Geometry: final body of the model. Coordinates: model frame, mm. A direction names the side the tool comes from. Coordinates: 2 decimals unless noted, no trailing zeros. Loops run counter-clockwise (first coordinate to the right, second up) from the corner with the lowest first, then second, coordinate; pieces in that order, holes last. Notation, with made-up numbers: (88, 66) - (136, 66) arc R22 ccw to (136, 78) - close; hole circle Ø2 at (0.5, 6.25). An arc over 180 degrees is marked (long way). Put each result on its own line as item: value. Start each with the question number.
1) Section B-B on y = 45. Output: boundary loops of the cut face in (x, z), and give its area (3 significant figures).
2) Reachability of faces 5 (the cylindrical face through (38.315, -4.574, 3.614)), 6 (the cylindrical face through (40.354, 82.574, 5.325)), 7 (the cylindrical face through (-34.14, 4.9, 5.07)) from +Z, -Z, +X, -X, +Y, -Y: full face, straight path, thin tool, end or side. Return the list, or none.
3) Contact query for a flat-ended pin moving along its axis: pin 1 Ø2.5 at (x, z) = (-38.89, 5) entering from +Y. Output: stop coordinate, or through.
4) Section C-C on x = 6. Output: boundary loops of the cut face in (y, z).
5) Section D-D on y = 2. Output: boundary loops of the cut face in (x, z).
6) Material intervals for line 1 along X through (y, z) = (64, 7.25); line 2 along X through (y, z) = (82.15, 5); line 3 along Y through (x, z) = (9, 3.75), sorted ascending. Write a range as from..to.
7) Draft query along Z for faces 1 (the cylindrical face through (-44.4, -5.43, 5.07)), 2 (the cylindrical face through (-38.315, 82.574, 3.614)), 3 (the cylindrical face through (13.07, 78.93, 6.5)), 4 (the flat face through (0, 76, 10)). Return one class per face: +Z half, -Z half, draft (parallel to the pull), parting line (faces both ways), or undercut.
8) Section A-A on z = 1.5. Count the separate pieces of the cut face and the enclosed holes in it, and give its area (3 significant figures).
```python
from build123d import *

# Parameters (mm, degrees)
SKETCH1_R           = 3.5
SKETCH1_W           = 70
SKETCH1_H           = 70
BOSS_EXTRUDE1_DEPTH = 10
FILLET3_R           = 2
SKETCH3_R           = 1.5
CUT_EXTRUDE2_DEPTH  = 90
CUT_EXTRUDE4_REACH  = 103.119
SKETCH5_R           = 1.5
CUT_EXTRUDE5_REACH  = 103.119
SKETCH6_R           = 1.5
FILLET5_R           = 3
CUT_EXTRUDE6_REACH  = 97.818
SKETCH7_R           = 1.5


with BuildPart() as part:
    # Sketch1 → Boss-Extrude1 (new body)
    with BuildSketch(Plane.XY):
        Polygon((45, -6), (-45, -6), (-45, 6), (-45, 72), (-45, 84), (45, 84), (45, 72), (45, 6), align=None)
        with Locations((-38.781438859, 0)):
            Circle(SKETCH1_R, mode=Mode.SUBTRACT)
        with Locations(Location((38.781438859, 0, 0), (0, 0, 180))):
            Circle(SKETCH1_R, mode=Mode.SUBTRACT)
        with Locations(Location((-38.781438859, 78, 0), (0, 0, 180))):
            Circle(SKETCH1_R, mode=Mode.SUBTRACT)
        with Locations((38.781438859, 78)):
            Circle(SKETCH1_R, mode=Mode.SUBTRACT)
        with Locations((0, 39)):
            Rectangle(SKETCH1_W, SKETCH1_H, mode=Mode.SUBTRACT)
    extrude(amount=BOSS_EXTRUDE1_DEPTH)

    # Fillet3
    fillet3_edges = [part.edges().sort_by_distance(p)[0] for p in [
        (-45, 84, 5),
        (45, 84, 5),
        (45, -6, 5),
        (-45, -6, 5),
    ]]
    fillet(fillet3_edges, radius=FILLET3_R)

    # Sketch3 → Cut-Extrude2 (cut)
    with BuildSketch(Plane.XZ.offset(6)):
        with Locations(Location((-13, 5, 0), (0, 0, 270))):
            Circle(SKETCH3_R)
        with Locations(Location((13, 5, 0), (0, 0, 270))):
            Circle(SKETCH3_R)
    extrude(amount=-CUT_EXTRUDE2_DEPTH, mode=Mode.SUBTRACT)

    # Sketch5 → Cut-Extrude4 (cut, up to next)
    with BuildSketch(Plane.XZ.offset(6), mode=Mode.PRIVATE) as cut_extrude4_sk1:
        with Locations(Location((-38.89, 5, 0), (0, 0, 270))):
            Circle(SKETCH5_R)
    cut_extrude4_tool1 = extrude(cut_extrude4_sk1.sketch, amount=-CUT_EXTRUDE4_REACH, mode=Mode.PRIVATE) & part.part
    # Sketch5 → Cut-Extrude4 (cut, up to next)
    with BuildSketch(Plane.XZ.offset(6), mode=Mode.PRIVATE) as cut_extrude4_sk2:
        with Locations(Location((38.89, 5, 0), (0, 0, 270))):
            Circle(SKETCH5_R)
    cut_extrude4_tool2 = extrude(cut_extrude4_sk2.sketch, amount=-CUT_EXTRUDE4_REACH, mode=Mode.PRIVATE) & part.part
    add(cut_extrude4_tool1.solids().sort_by_distance((-38.89, -6, 5))[0], mode=Mode.SUBTRACT)
    add(cut_extrude4_tool2.solids().sort_by_distance((38.89, -6, 5))[0], mode=Mode.SUBTRACT)

    # Sketch6 → Cut-Extrude5 (cut, up to next)
    with BuildSketch(Plane(origin=(0, 84, 0), x_dir=(1, 0, 0), z_dir=(0, 1, 0)), mode=Mode.PRIVATE) as cut_extrude5_sk1:
        with Locations(Location((-38.89, -5, 0), (0, 0, 90))):
            Circle(SKETCH6_R)
    cut_extrude5_tool1 = extrude(cut_extrude5_sk1.sketch, amount=-CUT_EXTRUDE5_REACH, mode=Mode.PRIVATE) & part.part
    # Sketch6 → Cut-Extrude5 (cut, up to next)
    with BuildSketch(Plane(origin=(0, 84, 0), x_dir=(1, 0, 0), z_dir=(0, 1, 0)), mode=Mode.PRIVATE) as cut_extrude5_sk2:
        with Locations(Location((38.89, -5, 0), (0, 0, 90))):
            Circle(SKETCH6_R)
    cut_extrude5_tool2 = extrude(cut_extrude5_sk2.sketch, amount=-CUT_EXTRUDE5_REACH, mode=Mode.PRIVATE) & part.part
    add(cut_extrude5_tool1.solids().sort_by_distance((-38.89, 84, 5))[0], mode=Mode.SUBTRACT)
    add(cut_extrude5_tool2.solids().sort_by_distance((38.89, 84, 5))[0], mode=Mode.SUBTRACT)

    # Fillet5
    fillet5_edges = [part.edges().sort_by_distance(p)[0] for p in [
        (-35, 74, 5),
        (-35, 4, 5),
        (35, 4, 5),
        (35, 74, 5),
    ]]
    fillet(fillet5_edges, radius=FILLET5_R)

    # Sketch7 → Cut-Extrude6 (cut, up to next)
    with BuildSketch(Plane.XY.offset(10), mode=Mode.PRIVATE) as cut_extrude6_sk1:
        with Locations((-25, 79)):
            Circle(SKETCH7_R)
    cut_extrude6_tool1 = extrude(cut_extrude6_sk1.sketch, amount=-CUT_EXTRUDE6_REACH, mode=Mode.PRIVATE) & part.part
    # Sketch7 → Cut-Extrude6 (cut, up to next)
    with BuildSketch(Plane.XY.offset(10), mode=Mode.PRIVATE) as cut_extrude6_sk2:
        with Locations(Location((25, 79, 0), (0, 0, 180))):
            Circle(SKETCH7_R)
    cut_extrude6_tool2 = extrude(cut_extrude6_sk2.sketch, amount=-CUT_EXTRUDE6_REACH, mode=Mode.PRIVATE) & part.part
    # Sketch7 → Cut-Extrude6 (cut, up to next)
    with BuildSketch(Plane.XY.offset(10), mode=Mode.PRIVATE) as cut_extrude6_sk3:
        with Locations((25, -1)):
            Circle(SKETCH7_R)
    cut_extrude6_tool3 = extrude(cut_extrude6_sk3.sketch, amount=-CUT_EXTRUDE6_REACH, mode=Mode.PRIVATE) & part.part
    # Sketch7 → Cut-Extrude6 (cut, up to next)
    with BuildSketch(Plane.XY.offset(10), mode=Mode.PRIVATE) as cut_extrude6_sk4:
        with Locations(Location((-25, -1, 0), (0, 0, 180))):
            Circle(SKETCH7_R)
    cut_extrude6_tool4 = extrude(cut_extrude6_sk4.sketch, amount=-CUT_EXTRUDE6_REACH, mode=Mode.PRIVATE) & part.part
    # Sketch7 → Cut-Extrude6 (cut, up to next)
    with BuildSketch(Plane.XY.offset(10), mode=Mode.PRIVATE) as cut_extrude6_sk5:
        with Locations((40, 64)):
            Circle(SKETCH7_R)
    cut_extrude6_tool5 = extrude(cut_extrude6_sk5.sketch, amount=-CUT_EXTRUDE6_REACH, mode=Mode.PRIVATE) & part.part
    # Sketch7 → Cut-Extrude6 (cut, up to next)
    with BuildSketch(Plane.XY.offset(10), mode=Mode.PRIVATE) as cut_extrude6_sk6:
        with Locations(Location((40, 14, 0), (0, 0, 180))):
            Circle(SKETCH7_R)
    cut_extrude6_tool6 = extrude(cut_extrude6_sk6.sketch, amount=-CUT_EXTRUDE6_REACH, mode=Mode.PRIVATE) & part.part
    # Sketch7 → Cut-Extrude6 (cut, up to next)
    with BuildSketch(Plane.XY.offset(10), mode=Mode.PRIVATE) as cut_extrude6_sk7:
        with Locations((-40, 14)):
            Circle(SKETCH7_R)
    cut_extrude6_tool7 = extrude(cut_extrude6_sk7.sketch, amount=-CUT_EXTRUDE6_REACH, mode=Mode.PRIVATE) & part.part
    # Sketch7 → Cut-Extrude6 (cut, up to next)
    with BuildSketch(Plane.XY.offset(10), mode=Mode.PRIVATE) as cut_extrude6_sk8:
        with Locations(Location((-40, 64, 0), (0, 0, 180))):
            Circle(SKETCH7_R)
    cut_extrude6_tool8 = extrude(cut_extrude6_sk8.sketch, amount=-CUT_EXTRUDE6_REACH, mode=Mode.PRIVATE) & part.part
    add(cut_extrude6_tool1.solids().sort_by_distance((-25, 79, 10))[0], mode=Mode.SUBTRACT)
    add(cut_extrude6_tool2.solids().sort_by_distance((25, 79, 10))[0], mode=Mode.SUBTRACT)
    add(cut_extrude6_tool3.solids().sort_by_distance((25, -1, 10))[0], mode=Mode.SUBTRACT)
    add(cut_extrude6_tool4.solids().sort_by_distance((-25, -1, 10))[0], mode=Mode.SUBTRACT)
    add(cut_extrude6_tool5.solids().sort_by_distance((40, 64, 10))[0], mode=Mode.SUBTRACT)
    add(cut_extrude6_tool6.solids().sort_by_distance((40, 14, 10))[0], mode=Mode.SUBTRACT)
    add(cut_extrude6_tool7.solids().sort_by_distance((-40, 14, 10))[0], mode=Mode.SUBTRACT)
    add(cut_extrude6_tool8.solids().sort_by_distance((-40, 64, 10))[0], mode=Mode.SUBTRACT)


solid = part.part
```
Answer block:
1. outline: (-45, 0) - (-35, 0) - (-35, 10) - (-45, 10) - close; (35, 0) - (45, 0) - (45, 10) - (35, 10) - close
1. area: 200 mm²
2. face 5: -Y
2. face 6: +Y
2. face 7: +Z, -Z
3. pin 1: stops at y = 74.77
4. outline: (-6, 0) - (4, 0) - (4, 10) - (-6, 10) - close; (74, 0) - (84, 0) - (84, 10) - (74, 10) - close
5. outline: (-45, 0) - (-41.65, 0) - (-41.65, 10) - (-45, 10) - close; (-35.91, 0) - (35.91, 0) - (35.91, 10) - (-35.91, 10) - close; (41.65, 0) - (45, 0) - (45, 10) - (41.65, 10) - close; hole circle Ø3 at (-13, 5); hole circle Ø3 at (13, 5)
6. line 1: x = -45..-41.5, -38.5..-35, 35..38.5, 41.5..45
6. line 2: x = -44.99..-40.39, -37.39..-14.5, -11.5..11.5, 14.5..37.39, 40.39..44.99
6. line 3: y = -6..4, 74..84
7. face 1: draft
7. face 2: undercut
7. face 3: undercut
7. face 4: +Z half
8. separate pieces: 1
8. enclosed holes: 13
8. area: 2,990 mm²
